Check sheet for the drawn part. Datum: minimum x, y, z corner. Units: mm. A direction names the side the tool comes from. Give positions to 0.01 mm unless a question says otherwise; leave off trailing zeros. Order: outer loops, then holes, each group sorted by start corner. A loop starts at its lowest first (then second) coordinate and runs counter-clockwise, first axis right, second up. Notation, with made-up numbers: (18, 88) - (62, 88) arc R13 cw to (62, 103) - close; hole circle Ø1 at (44, -32). An arc over 180 degrees is marked (long way). Answer as a JSON object with one key per item and string values. Group by question number.
(1) Access from +Z, -Z, +X, -X, +Y, -Y to the whole of each face (thin tool, end or side, straight path). Record for the marked faces 1 and 2.
(2) Thickness scan on line 1 (X direction, y = 23, z = 56); line 2 (Z direction, x = 4, y = 17.5); line 3 (X direction, y = 27.5, z = 45.5) (1 decimal). Record the ranges inside material, lowest first.
(3) Section check B-B (y = 7). Record the boundary of the cut face in (x, z), then the cut area to 3 significant figures.
(4) Depth check by flat-ended pin: pin 1 Ø1 at (y, z) = (32.5, 24) entering from -X (1 decimal); pin 2 Ø10 at (y, z) = (36.5, 34.5) entering from +X; pin 3 Ø8 at (x, y) = (7.5, 36) entering from -Z; pin 4 Ø12 at (y, z) = (15.5, 55.5) entering from +X. Enter the tip coordinate at first touch or a pass-through.
(5) Section check A-A (z = 18). Record the boundary of the cut face in (x, y) (1 decimal), then the cut area to 3 significant figures.
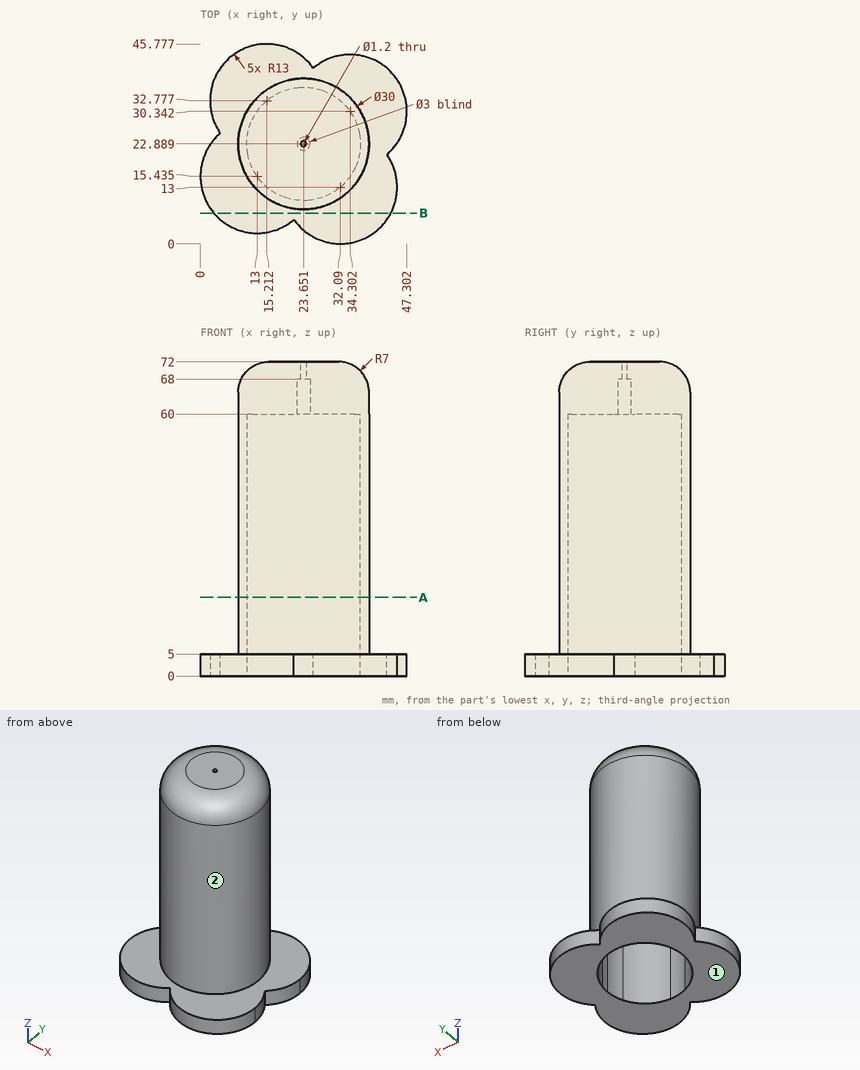
Solutions:
{
 "1": {"face 1": "-Z, +X, -X, +Y, -Y", "face 2": "+Z"},
 "2": {"line 1": "x = 8.65 to 10.65, 36.65 to 38.65", "line 2": "z = 0 to 5", "line 3": "x = 9.4 to 11.5, 35.8 to 37.9"},
 "3": {"outline": "(3.11, 0) - (43.62, 0) - (43.62, 5) - (3.11, 5) - close", "area": "203 mm2"},
 "4": {"pin 1": "stops at x = 11.7", "pin 2": "stops at x = 35.93", "pin 3": "stops at z = 0", "pin 4": "stops at x = 38.59"},
 "5": {"outline": "circle Ø30 at (23.7, 22.9); hole circle Ø26 at (23.7, 22.9)", "area": "176 mm2"}
}
